Can you work these out from the model? Positions are in its coordinate system, mm. A direction names the side the tool comes from. Round coordinates to 2 decimals unless told otherwise and drop trailing zeros. Write each loop counter-clockwise with the first axis right and the second up, starting at its lowest first coordinate (ties: lowest second). Pieces come first, ordered by that corner, then holes. Notation, with made-up numbers: (33, 29) -> (69, 29) arc R21 cw to (69, 41) -> close; hole circle Ø5 at (45, 59.25). An arc over 180 degrees is marked (long way). Write item = value, one per line. Start each with the question number.
1) Imagine slicing it at C-C, the plane x = -14.5. Please give me the cut outline in (y, z), then the cut area to 3 significant figures.
2) Thinking about a two-plate mould opening in Z: for faces 3 (the face through (15.67, 5.75, -23.27)), 4 (the face through (-10, 1, 13)), 5 (the face through (64.26, 5.75, 12.99)), which applies, +Z half, -Z half, draft (parallel to the pull), parting line (faces both ways), or undercut?
3) Imagine slicing it at A-A, the plane y = 3. Please give me the cut outline in (x, z).
4) I'm going to push flat-ended pins straight in: pin 1 (1 mm diameter, centred on y = 5, z = 3.5, fed in from +X); pin 2 (3 mm diameter, centred on x = -9, z = 14.5, fed in from +Y). Where does each tip first touch, or does it pass through?
5) If I drill on line 1 (X direction, y = 5.75, z = 10); line 2 (X direction, y = 5.25, z = 18); line 3 (Z direction, x = 19, y = 6), over which ranges is the centre line in solid material (lowest first)?
6) Imagine slicing it at B-B, the plane x = 4. Please give me the cut outline in (y, z).
7) For faces 1 (the face through (14, 2, 51.015)), 2 (the face through (0, 1.5, 13)), which set-ups out of +Z, -Z, +X, -X, +Y, -Y let a thin tool reach every point of the face, with its end or its side?
from build123d import *

# Parameters (mm, degrees)
SKETCH2_W           = 100
SKETCH2_H           = 75
BOSS_EXTRUDE1_DEPTH = 6.5
FILLET1_R           = 2.5
CUT_EXTRUDE1_DEPTH  = 5
FILLET3_R           = 6
SKETCH4_R           = 3.25
CUT_EXTRUDE2_DEPTH  = 0.5


with BuildPart() as part:
    # Sketch2 → Boss-Extrude1 (new body)
    with BuildSketch(Plane(origin=(0, 0, 0), x_dir=(1, 0, 0), z_dir=(0, 1, 0))):
        with Locations((14.972577697, -13.514625229)):
            Rectangle(SKETCH2_W, SKETCH2_H)
    extrude(amount=BOSS_EXTRUDE1_DEPTH)

    # Fillet1
    fillet1_edges = [part.edges().sort_by_distance(p)[0] for p in [
        (64.972577697, 6.5, 13.514625229),
        (14.972577697, 6.5, -23.985374771),
        (-35.027422303, 6.5, 13.514625229),
        (14.972577697, 6.5, 51.014625229),
    ]]
    fillet(fillet1_edges, radius=FILLET1_R)

    # Sketch3 → Cut-Extrude1 (cut)
    with BuildSketch(Plane(origin=(0, 6.5, 0), x_dir=(1, 0, 0), z_dir=(0, 1, 0))):
        with BuildLine():
            Line((-3.42616702, -9.514625229), (13.213071542, -9.514625229))
            ThreePointArc((13.213071542, -9.514625229), (17.213071542, -13.514625229), (13.213071542, -17.514625229))
            Line((13.213071542, -17.514625229), (-3.42616702, -17.514625229))
            ThreePointArc((-3.42616702, -17.514625229), (-17.70568068, -13.514625229), (-3.42616702, -9.514625229))
        make_face()
    extrude(amount=-CUT_EXTRUDE1_DEPTH, mode=Mode.SUBTRACT)

    # Fillet3
    fillet3_edges = [part.edges().sort_by_distance(p)[0] for p in [
        (-3.42616702, 4, 17.514625229),
        (-3.42616702, 4, 9.514625229),
    ]]
    fillet(fillet3_edges, radius=FILLET3_R)

    # Sketch4 → Cut-Extrude2 (cut)
    with BuildSketch(Plane(origin=(0, 1.5, 0), x_dir=(1, 0, 0), z_dir=(0, 1, 0))):
        with Locations(Location((-9.992086902, -13.532706959, 0), (0, 0, 270))):
            Circle(SKETCH4_R)
    extrude(amount=-CUT_EXTRUDE2_DEPTH, mode=Mode.SUBTRACT)


solid = part.part
Reported:
q1.outline = (0, -23.99) -> (4, -23.99) arc R2.5 ccw to (6.5, -21.49) -> (6.5, 7.26) -> (1.5, 7.26) -> (1.5, 19.77) -> (6.5, 19.77) -> (6.5, 48.51) arc R2.5 ccw to (4, 51.01) -> (0, 51.01) -> close
q1.area = 422 mm²
q2.face_3 = -Z half
q2.face_4 = undercut
q2.face_5 = draft
q3.outline = (-35.03, -23.99) -> (64.97, -23.99) -> (64.97, 51.01) -> (-35.03, 51.01) -> close; hole (-4.74, 7.89) arc R6 cw to (-0.64, 9.51) -> (13.21, 9.51) arc R4 ccw to (13.21, 17.51) -> (-0.64, 17.51) arc R6 cw to (-4.74, 19.14) arc R7.7 ccw (long way) to start
q4.pin_1 = 64.92
q4.pin_2 = 1
q5.line_1 = -34.31 to -16.86, 15.12 to 64.26
q5.line_2 = -34.69 to -16.26, -3.01 to 64.64
q5.line_3 = -22.99 to 50.01
q6.outline = (0, -23.99) -> (4, -23.99) arc R2.5 ccw to (6.5, -21.49) -> (6.5, 9.51) -> (1.5, 9.51) -> (1.5, 17.51) -> (6.5, 17.51) -> (6.5, 48.51) arc R2.5 ccw to (4, 51.01) -> (0, 51.01) -> close
q7.face_1 = +Z, +X, -X, +Y, -Y
q7.face_2 = +Y
